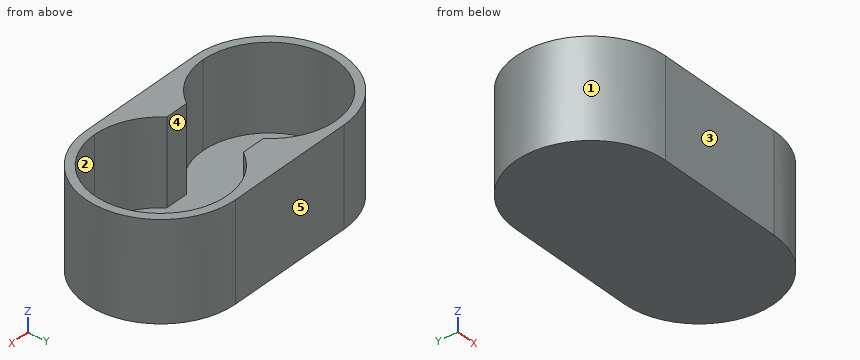
Autodesk Inventor part; units mm, degrees
ref_plane "YZ Plane" through (0, 0, 0) normal (1, 0, 0) x (0, 1, 0)
ref_plane "XZ Plane" through (0, 0, 0) normal (0, 1, 0) x (-1, 0, 0)
ref_plane "XY Plane" through (0, 0, 0) normal (0, 0, 1) x (1, 0, 0)
sketch "スケッチ1" plane through (0, 0, 0) normal (0, 0, 1) x (1, 0, 0)
  arc A0 (7.8, -7.8) -> (7.8, 7.8) centre (7.8, 0) ccw
  arc A1 (-7.8, 7.8) -> (-7.8, -7.8) centre (-7.8, 0) ccw
  line L0 (-7.8, 7.8) -> (7.8, 7.8)
  line L1 (7.8, -7.8) -> (-7.8, -7.8)
  line L2 (7.8, 8.8) -> (-7.8, 8.8)
  arc A2 (-7.8, 8.8) -> (-7.8, -8.8) centre (-7.8, 0) ccw
  line L3 (-7.8, -8.8) -> (7.8, -8.8)
  arc A3 (7.8, -8.8) -> (7.8, 8.8) centre (7.8, 0) ccw
  point P0 (0, 0)
  dimension "d0" = 15.6
  dimension "d1" = 15.6
  dimension "d2" = 7.8
  dimension "d3" = 1
extrude "押し出し1" add sketch "スケッチ1" along normal blind 10
sketch "スケッチ2" plane through (0, 0, 0) normal (0, 0, -1) x (-1, 0, 0)
  line L0 (-7.8, 7.8) -> (7.8, 7.8)
  arc A0 (7.8, -7.8) -> (7.8, 7.8) centre (7.8, 0) ccw
  line L1 (7.8, -7.8) -> (-7.8, -7.8)
  arc A1 (-7.8, 7.8) -> (-7.8, -7.8) centre (-7.8, 0) ccw
  line L2 (-7.8, 8.8) -> (7.8, 8.8)
  arc A2 (-7.8, 8.8) -> (-7.8, -8.8) centre (-7.8, 0) ccw
  line L3 (7.8, -8.8) -> (-7.8, -8.8)
  arc A3 (7.8, -8.8) -> (7.8, 8.8) centre (7.8, 0) ccw
  point P0 (0, 0)
extrude "押し出し2" add sketch "スケッチ2" along normal blind 1.5 contours L0 A0 L1 A1 | L2 A3 L3 A2
sketch "スケッチ3" plane through (0, 0, 0) normal (0, 0, 1) x (1, 0, 0)
  arc A0 (-7.8, 7.8) -> (-7.8, -7.8) centre (-7.8, 0) ccw
  arc A1 (-7.8, -7.8) -> (-1.429, -4.5) centre (-7.8, 0) ccw
  arc A2 (7.8, -7.8) -> (7.8, 7.8) centre (7.8, 0) ccw
  arc A3 (1.429, -4.5) -> (7.8, -7.8) centre (7.8, 0) ccw
  line L0 (-1.429, -4.5) -> (1.429, -4.5)
  line L1 (7.8, -7.8) -> (-7.8, -7.8)
  line L2 (-7.8, -7.8) -> (7.8, -7.8)
  arc A4 (-1.429, 4.5) -> (-7.8, 7.8) centre (-7.8, 0) ccw
  arc A5 (7.8, 7.8) -> (1.429, 4.5) centre (7.8, 0) ccw
  line L3 (-1.429, 4.5) -> (1.429, 4.5)
  line L4 (-7.8, 7.8) -> (7.8, 7.8)
  line L5 (7.8, 7.8) -> (-7.8, 7.8)
  point P0 (0, 0)
  dimension "d9" = 9
extrude "押し出し3" add sketch "スケッチ3" along normal up to surface (10 mm away) contours L4 A5 L3 A4 | A1 L0 A3 L1
properties part number "CaseBottom_CR123A"
Source: CAD feature listing. Evaluate the final solid. Frame: model axes, mm. Face numbers are marked on the shaded views. A direction names the side the tool comes from. Coordinates: 2 decimals unless noted, no trailing zeros. Loops run counter-clockwise (first coordinate to the right, second up) from the corner with the lowest first, then second, coordinate; pieces in that order, holes last. Notation, with made-up numbers: M 44.25,40.25 L 69.25,40.25 A27 cw 69.25,66.25 Z; hole C 36.25,-3 d8. An arc over 180 degrees is marked long. Use CSV: the item, a comma, the result in double quotes.
(1) Cut plane A-A on z = 8.25. Return loops of the section in (x, y), and give its area (3 significant figures).
Answers follow:
outline,"M -7.8,-8.8 L 7.8,-8.8 A8.8 ccw 7.8,8.8 L -7.8,8.8 A8.8 ccw Z; hole M -7.8,-7.8 A7.8 ccw -1.43,-4.5 L 1.43,-4.5 A7.8 ccw 7.8,-7.8 A7.8 ccw 7.8,7.8 A7.8 ccw 1.43,4.5 L -1.43,4.5 A7.8 ccw -7.8,7.8 A7.8 ccw Z"
area,"127 mm²"
(2) Reachability of the marked faces 4 and 5 from +Z, -Z, +X, -X, +Y, -Y: full face, straight path, thin tool, end or side. Return the list, or none.
Answers follow:
face 4,"+Z"
face 5,"+Z, -Z, +X, -X, +Y"
(3) Cut plane C-C on x = 6.5. Return loops of the section in (y, z).
Answers follow:
outline,"M -8.8,-1.5 L 8.8,-1.5 L 8.8,10 L 7.69,10 L 7.69,0 L -7.69,0 L -7.69,10 L -8.8,10 Z"
(4) Cut plane B-B on y = 0. Return loops of the section in (x, z), and give its area (3 significant figures).
Answers follow:
outline,"M -16.6,-1.5 L 16.6,-1.5 L 16.6,10 L 15.6,10 L 15.6,0 L -15.6,0 L -15.6,10 L -16.6,10 Z"
area,"69.8 mm²"
(5) Draft query along X for the marked faces 1, 2 and 3. Return one class per face: pulls with the +X half, pulls with the -X half, needs draft (parallel to the pull), parting line crosses it, or undercut.
Answers follow:
face 1,"pulls with the -X half"
face 2,"undercut"
face 3,"needs draft"
(6) Contact query for flat-ended pins moving along their axis: pin 1 (3 mm diameter, centred on y = -3, z = 2.5, fed in from +X); pin 2 (1 mm diameter, centred on x = 11, z = 6, fed in from -Y); pin 3 (3 mm diameter, centred on x = -10.5, y = 3.5, fed in from +Z). Output: stop coordinate, or through.
Answers follow:
pin 1,"x = 16.47"
pin 2,"y = -8.38"
pin 3,"z = 0"
(7) Cut plane D-D on y = -6. Return loops of the section in (x, z).
Answers follow:
outline,"M -14.24,-1.5 L 14.24,-1.5 L 14.24,10 L 12.78,10 L 12.78,0 L 2.82,0 L 2.82,10 L -2.82,10 L -2.82,0 L -12.78,0 L -12.78,10 L -14.24,10 Z"
(8) Line query: line 1 (X direction, y = -0.25, z = 6.25); line 2 (X direction, y = 6, z = 8); line 3 (Z direction, x = -12.5, y = -4.5). Output: solid intervals per line, ascending. Write a range as [from, to].
Answers follow:
line 1,"[-16.6, -15.6], [15.6, 16.6]"
line 2,"[-14.24, -12.78], [-2.82, 2.82], [12.78, 14.24]"
line 3,"[-1.5, 0]"
